from build123d import *

# Parameters (mm, degrees)
SKETCH1_W           = 63.5
SKETCH1_H           = 50.8
BOSS_EXTRUDE1_DEPTH = 25.4
SKETCH3_W           = 44.45
SKETCH3_H           = 43.18
CUT_EXTRUDE1_DEPTH  = 38.1
SKETCH5_R           = 4.826
CUT_EXTRUDE2_DEPTH  = 76.2
FILLET3_R           = 1.27
SKETCH10_W          = 12.7
SKETCH10_H          = 2.54
BOSS_EXTRUDE4_DEPTH = 7.62
SKETCH11_W          = 12.7
SKETCH11_H          = 2.54
BOSS_EXTRUDE5_DEPTH = 7.62
CUT_EXTRUDE5_REACH  = 91.262
SKETCH12_R          = 3.175
SKETCH13_W          = 5.08
SKETCH13_H          = 5.08
BOSS_EXTRUDE6_DEPTH = 6.35
CUT_EXTRUDE6_REACH  = 83.876
SKETCH15_R          = 1.905
FILLET5_R           = 2.54


with BuildPart() as part:
    # Sketch1 → Boss-Extrude1 (new body)
    with BuildSketch(Plane.XY):
        with Locations((31.75, 25.4)):
            Rectangle(SKETCH1_W, SKETCH1_H)
    extrude(amount=BOSS_EXTRUDE1_DEPTH)

    # Sketch3 → Cut-Extrude1 (cut)
    with BuildSketch(Plane(origin=(0, 0, 0), x_dir=(-1, 0, 0), z_dir=(0, 0, -1))):
        with Locations((-41.275, 25.4)):
            Rectangle(SKETCH3_W, SKETCH3_H)
    extrude(amount=-CUT_EXTRUDE1_DEPTH, mode=Mode.SUBTRACT)

    # Sketch5 → Cut-Extrude2 (cut)
    with BuildSketch(Plane.XZ):
        with Locations(Location((44.45, 12.7, 0), (0, 0, 270))):
            Circle(SKETCH5_R)
    extrude(amount=-CUT_EXTRUDE2_DEPTH, mode=Mode.SUBTRACT)

    # Fillet3
    fillet3_edges = [part.edges().sort_by_distance(p)[0] for p in [
        (63.5, 3.81, 12.7),
        (63.5, 46.99, 12.7),
        (19.05, 46.99, 12.7),
        (19.05, 3.81, 12.7),
        (0, 50.8, 12.7),
        (63.5, 50.8, 12.7),
        (63.5, 0, 12.7),
        (0, 0, 12.7),
    ]]
    fillet(fillet3_edges, radius=FILLET3_R)

    # Sketch10 → Boss-Extrude4 (add)
    with BuildSketch(Plane.XZ):
        with Locations((31.75, 1.27)):
            Rectangle(SKETCH10_W, SKETCH10_H)
    extrude(amount=BOSS_EXTRUDE4_DEPTH)

    # Sketch11 → Boss-Extrude5 (add)
    with BuildSketch(Plane(origin=(0, 50.8, 0), x_dir=(1, 0, 0), z_dir=(0, 1, 0))):
        with Locations((31.75, -1.27)):
            Rectangle(SKETCH11_W, SKETCH11_H)
    extrude(amount=BOSS_EXTRUDE5_DEPTH)

    # Sketch12 → Cut-Extrude5 (cut, up to next)
    with BuildSketch(Plane.XY.offset(2.54), mode=Mode.PRIVATE) as cut_extrude5_sk1:
        with Locations((31.75, 54.61)):
            Circle(SKETCH12_R)
    cut_extrude5_tool1 = extrude(cut_extrude5_sk1.sketch, amount=-CUT_EXTRUDE5_REACH, mode=Mode.PRIVATE) & part.part
    # Sketch12 → Cut-Extrude5 (cut, up to next)
    with BuildSketch(Plane.XY.offset(2.54), mode=Mode.PRIVATE) as cut_extrude5_sk2:
        with Locations((31.75, -3.81)):
            Circle(SKETCH12_R)
    cut_extrude5_tool2 = extrude(cut_extrude5_sk2.sketch, amount=-CUT_EXTRUDE5_REACH, mode=Mode.PRIVATE) & part.part
    add(cut_extrude5_tool1.solids().sort_by_distance((31.75, 54.61, 2.54))[0], mode=Mode.SUBTRACT)
    add(cut_extrude5_tool2.solids().sort_by_distance((31.75, -3.81, 2.54))[0], mode=Mode.SUBTRACT)

    # Sketch13 → Boss-Extrude6 (add)
    with BuildSketch(Plane(origin=(0, 0, 0), x_dir=(-1, 0, 0), z_dir=(0, 0, -1))):
        with Locations((-9.525, 25.4)):
            Rectangle(SKETCH13_W, SKETCH13_H)
    extrude(amount=BOSS_EXTRUDE6_DEPTH)

    # Sketch15 → Cut-Extrude6 (cut, up to next)
    with BuildSketch(Plane(origin=(12.065, 0, 0), x_dir=(0, 0, -1), z_dir=(1, 0, 0)), mode=Mode.PRIVATE) as cut_extrude6_sk1:
        with Locations((3.175, 25.4)):
            Circle(SKETCH15_R)
    cut_extrude6_tool1 = extrude(cut_extrude6_sk1.sketch, amount=-CUT_EXTRUDE6_REACH, mode=Mode.PRIVATE) & part.part
    add(cut_extrude6_tool1.solids().sort_by_distance((12.065, 25.4, -3.175))[0], mode=Mode.SUBTRACT)

    # Fillet5
    fillet5_edges = [part.edges().sort_by_distance(p)[0] for p in [
        (9.525, 27.94, -6.35),
        (9.525, 22.86, -6.35),
    ]]
    fillet(fillet5_edges, radius=FILLET5_R - 0.0001)  # a hair under: the kernel refuses the full size


solid = part.part
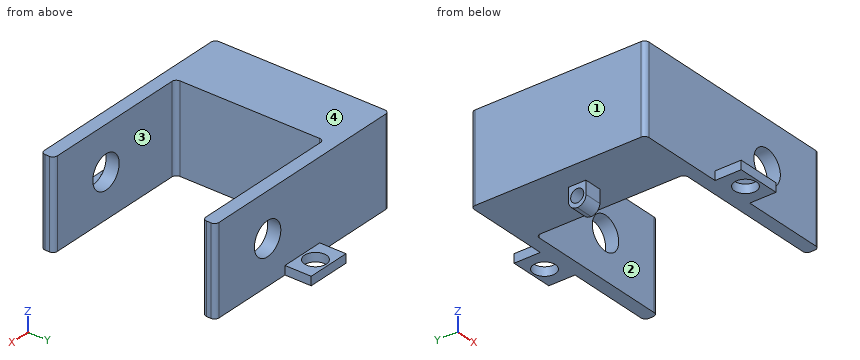
Geometry check sheet. Reference: the model listing, model coordinates, mm. Face numbers are marked on the shaded views. A direction names the side the tool comes from. Give positions to 0.01 mm unless a question says otherwise; leave off trailing zeros. Order: outer loops, then holes, each group sorted by start corner. A loop starts at its lowest first (then second) coordinate and runs counter-clockwise, first axis right, second up. Notation, with made-up numbers: (-2.75, -5) - (28.25, -5) arc R17 ccw to (28.25, 23) - close; hole circle Ø6 at (-34, 85.25). An arc over 180 degrees is marked (long way). Answer as a JSON object with one key per item and string values.
(1) Material ranges on line 1 (Y direction, x = 22.5, z = 5.5); line 2 (Y direction, x = 31, z = 1); line 3 (X direction, y = 48.6, z = 12.7), recorded low to high.
Report:
{"line 1": "0 to 3.81, 46.99 to 50.8", "line 2": "-7.62 to -6.9, -0.72 to 3.81, 46.99 to 51.52, 57.7 to 58.42", "line 3": "0 to 39.62, 49.28 to 63.5"}
(2) Draft check along Y on the marked faces 1 and 2. Enter one of: released by +Y, released by -Y, zero draft, split by the parting line, or undercut.
Report:
{"face 1": "zero draft", "face 2": "undercut"}
(3) Depth check by flat-ended pin: pin 1 Ø19 at (x, y) = (21, 15) entering from -Z; pin 2 Ø3.5 at (y, z) = (25.4, -3.175) entering from -X; pin 3 Ø3 at (y, z) = (56.5, 1) entering from +X; pin 4 Ø15.5 at (x, z) = (44.45, 12.7) entering from -Y. Enter the tip coordinate at first touch or a pass-through.
Report:
{"pin 1": "z = 0", "pin 2": "through", "pin 3": "x = 38.1", "pin 4": "y = 0"}
(4) Tool access check on the marked faces 3 and 4. Record the directions out of +Z, -Z, +X, -X, +Y, -Y that give a thin tool (end or side, any length) a straight path to the whole face; none if there is none.
Report:
{"face 3": "+Z, -Z, +X", "face 4": "+Z, +X, -X, +Y, -Y"}
(5) Cross-section at B-B (z = 12.7). Record the cut outline in (x, y), then the cut area to 3 significant figures.
Report:
{"outline": "(0, 1.27) arc R1.27 ccw to (1.27, 0) - (39.62, 0) - (39.62, 3.81) - (20.32, 3.81) arc R1.27 cw to (19.05, 5.08) - (19.05, 45.72) arc R1.27 cw to (20.32, 46.99) - (39.62, 46.99) - (39.62, 50.8) - (1.27, 50.8) arc R1.27 ccw to (0, 49.53) - close; (49.28, 0) - (62.23, 0) arc R1.27 ccw to (63.5, 1.27) - (63.5, 2.54) arc R1.27 ccw to (62.23, 3.81) - (49.28, 3.81) - close; (49.28, 46.99) - (62.23, 46.99) arc R1.27 ccw to (63.5, 48.26) - (63.5, 49.53) arc R1.27 ccw to (62.23, 50.8) - (49.28, 50.8) - close", "area": "1,230 mm^2"}
(6) Cross-section at A-A (y = -3.81). Record the cut outline in (x, z) (3 decimals), then the cut area to 3 significant figures.
Report:
{"outline": "(25.4, 0) - (28.575, 0) - (28.575, 2.54) - (25.4, 2.54) - close; (34.925, 0) - (38.1, 0) - (38.1, 2.54) - (34.925, 2.54) - close", "area": "16.1 mm^2"}
(7) Cross-section at C-C (x = 36). Record the cut outline in (y, z), then the cut area to 3 significant figures.
Report:
{"outline": "(-7.62, 0) - (3.81, 0) - (3.81, 25.4) - (0, 25.4) - (0, 2.54) - (-7.62, 2.54) - close; (46.99, 0) - (58.42, 0) - (58.42, 2.54) - (50.8, 2.54) - (50.8, 25.4) - (46.99, 25.4) - close", "area": "232 mm^2"}
